The drawing under review shows one solid part. Ordinate dimensions are in mm from its lowest x, y, z. Round coordinates to 2 decimals unless told otherwise and drop trailing zeros. Order: outer loops, then holes, each group sorted by start corner. A loop starts at its lowest first (then second) coordinate and runs counter-clockwise, first axis right, second up.
1) To check wall thickness, follow L1, parallel to Y at x = 6, z = 9.5; L2, parallel to X at y = 6.5, z = 8.25; L3, parallel to X at y = 7, z = 7.25. State the ranges of each line that lie inside material, in increasing order.
2) Mouldability with a two-part tool opening along Y and no side actions: class the marked faces 1, 2 and 3 as pulls with the +Y half, pulls with the -Y half, needs draft (parallel to the pull), parting line crosses it, or undercut.
3) Consider section D-D (z = 13.75). Give the boundary of the cut face in (x, y).
4) Clearance check with a flat-ended pin moving along its axis: P1, Ø5, axis at x = 6, y = 7.5, coming from the -Z side. State where the tip first meets the part, or that it passes through.
5) Consider section A-A (y = 7.5). Give the boundary of the cut face in (x, z).
6) Consider section B-B (z = 7.25). Give the boundary of the cut face in (x, y).
7) Consider section C-C (x = 36). Give the boundary of the cut face in (y, z).
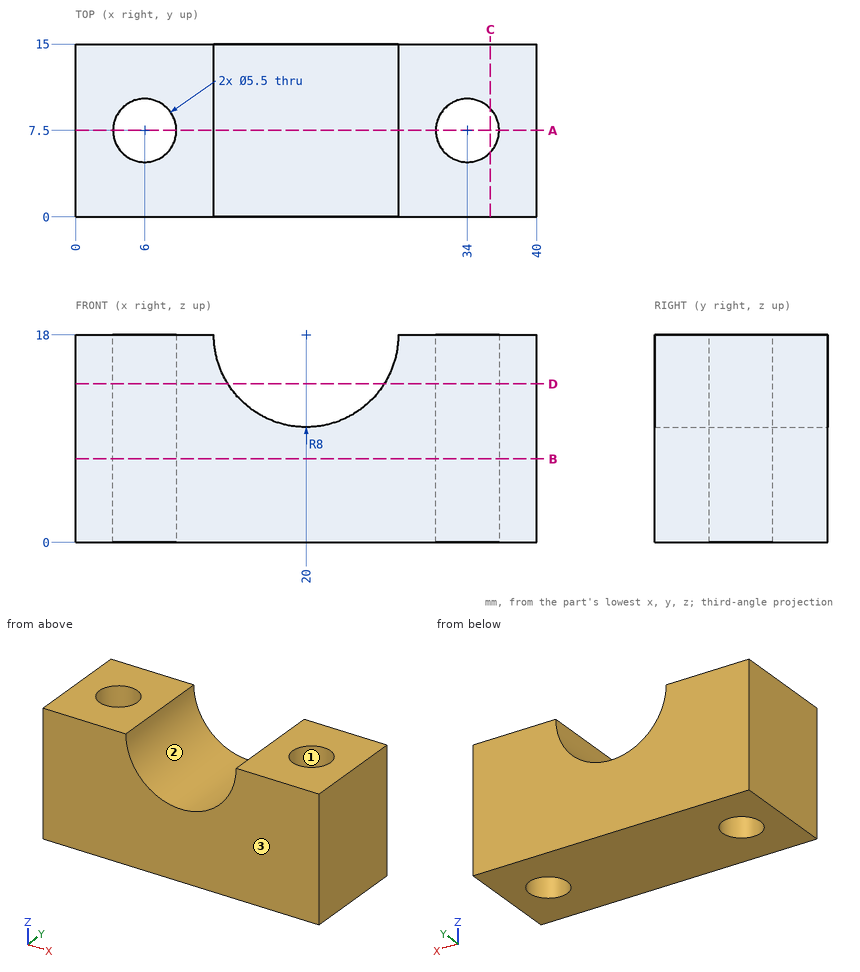
Answer below:
1. L1: y = 0 to 4.75, 10.25 to 15
1. L2: x = 0 to 3.44, 8.56 to 31.44, 36.56 to 40
1. L3: x = 0 to 3.3, 8.7 to 31.3, 36.7 to 40
2. face 1: undercut
2. face 2: needs draft
2. face 3: pulls with the -Y half
3. outline: (0, 0) - (13.22, 0) - (13.22, 15) - (0, 15) - close; (26.78, 0) - (40, 0) - (40, 15) - (26.78, 15) - close; hole circle Ø5.5 at (6, 7.5); hole circle Ø5.5 at (34, 7.5)
4. P1: passes through
5. outline: (0, 0) - (3.25, 0) - (3.25, 18) - (0, 18) - close; (8.75, 0) - (31.25, 0) - (31.25, 18) - (28, 18) arc R8 cw to (12, 18) - (8.75, 18) - close; (36.75, 0) - (40, 0) - (40, 18) - (36.75, 18) - close
6. outline: (0, 0) - (40, 0) - (40, 15) - (0, 15) - close; hole circle Ø5.5 at (6, 7.5); hole circle Ø5.5 at (34, 7.5)
7. outline: (0, 0) - (5.61, 0) - (5.61, 18) - (0, 18) - close; (9.39, 0) - (15, 0) - (15, 18) - (9.39, 18) - close
